Input: part model. Units: mm. Frame: model coordinates. A direction names the side the tool comes from. Coordinates: 2 decimals unless noted, no trailing zeros. Loops run counter-clockwise (first coordinate to the right, second up) from the corner with the lowest first, then second, coordinate; pieces in that order, holes last. Notation, with made-up numbers: M 17.5,-26.5 L 42.5,-26.5 A32 cw 42.5,7.5 Z; hole C -19.5,-34.5 d11. An arc over 180 degrees is marked long. Use a Markdown table: item, result. Add a question column.
1. Draft query along Z for faces 3 (the flat face through (10, -7, 0)), 4 (the flat face through (10, -5, 13)), 5 (the flat face through (10, -7, 10)). Return one class per face: +Z half, -Z half, draft (parallel to the pull), parting line (faces both ways), or undercut.
2. Section B-B on z = 11. Output: boundary loops of the cut face in (x, y), then the cut area to 3 significant figures.
3. Section C-C on y = -7.5. Output: boundary loops of the cut face in (x, z), then the cut area to 3 significant figures.
4. Set-up query: faces 1 (the flat face through (10, -15, 3)), 2 (the flat face through (10, -12, 5)). Return all of +Z, -Z, +X, -X, +Y, -Y with unobstructed straight access to the full face (end or side cutting, diameter ignored); none if empty.
5. Line query: L1, parallel to Y at x = 18, z = 5.75; L2, parallel to Z at x = 16.75, y = -8; L3, parallel to Z at x = 6.5, y = -10.75. Output: solid intervals per line, ascending. Write a range as [from, to].
6. Pin query (flat end, axial travel): pin 1 (2 mm diameter, centred on y = -12, z = 7.5, fed in from -X); pin 2 (1 mm diameter, centred on x = 2, y = -9, fed in from +Z); pin 3 (1.5 mm diameter, centred on x = 7.5, z = 12.5, fed in from -Y); pin 4 (4 mm diameter, centred on x = 6.5, z = 11.5, fed in from -Y). Return the tip coordinate at first contact, or that it passes through.
7. Section A-A on x = 4. Output: boundary loops of the cut face in (y, z), then the cut area to 3 significant figures.
```python
from build123d import *

# Parameters (mm, degrees)
F0_W     = 20
F0_H     = 5
F1_DEPTH = 15
F2_DEPTH = 10
F3_DEPTH = 5


with BuildPart() as f1:
    # F0 (on Front) → F1 (new body)
    with BuildSketch(Plane.XZ):
        with Locations((10, 2.5)):
            Rectangle(F0_W, F0_H)
    extrude(amount=F1_DEPTH)

    # F0 (on Front) → F2 (join)
    with BuildSketch(Plane.XZ):
        with Locations((10, 7.5)):
            Rectangle(F0_W, F0_H)
    extrude(amount=F2_DEPTH)

    # F0 (on Front) → F3 (join)
    with BuildSketch(Plane.XZ):
        with Locations((10, 12.5)):
            Rectangle(F0_W, F0_H)
    extrude(amount=F3_DEPTH)


solid = f1.part
```
Answers below:
| question | item | result |
|---|---|---|
| 1 | face 3 | -Z half |
| 1 | face 4 | draft |
| 1 | face 5 | +Z half |
| 2 | outline | M 0,-5 L 20,-5 L 20,0 L 0,0 Z |
| 2 | area | 100 mm² |
| 3 | outline | M 0,0 L 20,0 L 20,10 L 0,10 Z |
| 3 | area | 200 mm² |
| 4 | face 1 | +Z, -Z, +X, -X, -Y |
| 4 | face 2 | +Z, +X, -X, -Y |
| 5 | L1 | y = [-10, 0] |
| 5 | L2 | z = [0, 10] |
| 5 | L3 | z = [0, 5] |
| 6 | pin 1 | passes through |
| 6 | pin 2 | stops at z = 10 |
| 6 | pin 3 | stops at y = -5 |
| 6 | pin 4 | stops at y = -10 |
| 7 | outline | M -15,0 L 0,0 L 0,15 L -5,15 L -5,10 L -10,10 L -10,5 L -15,5 Z |
| 7 | area | 150 mm² |
